The model under review builds one solid part; all positions refer to its coordinate system, in mm. A direction names the side the tool comes from. Coordinates: 2 decimals unless noted, no trailing zeros. Order: outer loops, then holes, each group sorted by start corner. A loop starts at its lowest first (then second) coordinate and runs counter-clockwise, first axis right, second up. Notation, with made-up numbers: M 40.5,12 L 71.5,12 A35 cw 71.5,47 Z; hole C -37,80.25 d7. An arc over 180 degrees is marked long. One line per item, written item: value.
```python
from build123d import *

# Parameters (mm, degrees)
SKETCH_1_W                = 260
SKETCH_1_H                = 220
EXTRUDE_1_DEPTH           = 6
SKETCH_4_W                = 132
SKETCH_4_H                = 134
CUT_EXTRUDE_1_DEPTH       = 171.716138663
HOLE_WIZARD_1_D           = 6.6
HOLE_WIZARD_1_CBORE_D     = 11
HOLE_WIZARD_1_CBORE_DEPTH = 6.8
HOLE_WIZARD_M12_1_D       = 12
CUT_EXTRUDE_2_DEPTH       = 171.716138663
HOLE_WIZARD_M6_1_D        = 5
HOLE_WIZARD_M6_1_DEPTH    = 15
HOLE_WIZARD_M6_1_TIP      = 1.502151548
HOLE_WIZARD_3_D           = 6.6
HOLE_WIZARD_3_CBORE_D     = 11
HOLE_WIZARD_3_CBORE_DEPTH = 87
HOLE_WIZARD_2_D           = 6.6
HOLE_WIZARD_2_CBORE_D     = 11
HOLE_WIZARD_2_CBORE_DEPTH = 48
HOLE_WIZARD_1_2_D         = 4
HOLE_WIZARD_M4_1_D        = 3.3
HOLE_WIZARD_M4_1_DEPTH    = 10.1
HOLE_WIZARD_M4_1_TIP      = 0.991420021
HOLE_WIZARD_M4_2_D        = 3.3
HOLE_WIZARD_M4_2_DEPTH    = 10.1
HOLE_WIZARD_M4_2_TIP      = 0.991420021
CHAMFER_1_SIZE            = 30
FILLET_1_R                = 2


with BuildPart() as part:
    # 草图1 → 凸台-拉伸1 (new, symmetric)
    with BuildSketch(Plane(origin=(0, 0, 0), x_dir=(0, 0, -1), z_dir=(1, 0, 0))):
        Rectangle(SKETCH_1_W, SKETCH_1_H)
    extrude(amount=EXTRUDE_1_DEPTH, both=True)

    # 草图4 → 切除-拉伸1 (cut, through all)
    with BuildSketch(Plane(origin=(6, 0, 0), x_dir=(0, 0, -1), z_dir=(1, 0, 0))):
        with Locations((64, -43)):
            Rectangle(SKETCH_4_W, SKETCH_4_H)
    extrude(amount=-CUT_EXTRUDE_1_DEPTH, mode=Mode.SUBTRACT)

    # Hole Wizard 1 (through all)
    with Locations(Plane(origin=(-6, -19.944864322, 4.622627096), x_dir=(0, 0, -1), z_dir=(-1, 0, 0))):
        with Locations((8.622627096, -106.944864322), (8.622627096, -66.944864322)):
            CounterBoreHole(HOLE_WIZARD_1_D / 2, HOLE_WIZARD_1_CBORE_D / 2, HOLE_WIZARD_1_CBORE_DEPTH)

    # M12 间隙孔1 (through all)
    with Locations(Plane.ZY.offset(6)):
        with Locations((102, 90)):
            Hole(HOLE_WIZARD_M12_1_D / 2)

    # 草图7 → 切除-拉伸2 (cut, through all)
    with BuildSketch(Plane.ZY.offset(6)):
        with BuildLine():
            ThreePointArc((86.666512802, 17.861614446), (96.21364169, 16.477346637), (105.859776773, 16.351071812))
            ThreePointArc((105.859776773, 16.351071812), (112.428311092, 10.436736946), (106.513976226, 3.868202627))
            ThreePointArc((106.513976226, 3.868202627), (95.232902993, 4.015879966), (84.067616667, 5.634769437))
            ThreePointArc((84.067616667, 5.634769437), (79.25364223, 13.047640009), (86.666512802, 17.861614446))
        make_face()
        with BuildLine():
            ThreePointArc((67.434681402, -72.617038622), (88.956175335, -75.737506733), (110.700852725, -76.022160153))
            ThreePointArc((110.700852725, -76.022160153), (116.615187591, -69.453625834), (110.046653272, -63.539290969))
            ThreePointArc((110.046653272, -63.539290969), (89.936914032, -63.276040061), (70.033577537, -60.390193613))
            ThreePointArc((70.033577537, -60.390193613), (62.620706965, -65.20416805), (67.434681402, -72.617038622))
        make_face()
    extrude(amount=-CUT_EXTRUDE_2_DEPTH, mode=Mode.SUBTRACT)

    # M6 螺纹孔1
    with Locations(Plane(origin=(0, 0, -130), x_dir=(-1, 0, 0), z_dir=(0, 0, -1))):
        with Locations((0, 87), (0, 47)):
            Hole(HOLE_WIZARD_M6_1_D / 2, depth=HOLE_WIZARD_M6_1_DEPTH)
            with Locations((0, 0, -(HOLE_WIZARD_M6_1_DEPTH + HOLE_WIZARD_M6_1_TIP / 2))):  # 118° drill point
                Cone(0, HOLE_WIZARD_M6_1_D / 2, HOLE_WIZARD_M6_1_TIP, mode=Mode.SUBTRACT)

    # 打孔尺寸根据内六角圆柱头螺钉的类型3 (through all)
    with Locations(Plane(origin=(4.643601276, 65.309968696, 130), x_dir=(-1, 0, 0), z_dir=(0, 0, 1))):
        with Locations((4.643601276, 75.309968696), (4.643601276, 165.309968696)):
            CounterBoreHole(HOLE_WIZARD_3_D / 2, HOLE_WIZARD_3_CBORE_D / 2, HOLE_WIZARD_3_CBORE_DEPTH)

    # 打孔尺寸根据内六角圆柱头螺钉的类型2 (through all)
    with Locations(Plane(origin=(-2.196087781, 110, 22.857251804), x_dir=(-1, 0, 0), z_dir=(0, 1, 0))):
        with Locations((-2.196087781, -52.857251804), (-2.196087781, -132.857251804)):
            CounterBoreHole(HOLE_WIZARD_2_D / 2, HOLE_WIZARD_2_CBORE_D / 2, HOLE_WIZARD_2_CBORE_DEPTH)

    # Hole Wizard 1 2 (through all)
    with Locations(Plane.ZY.offset(6)):
        with Locations((2, 24)):
            Hole(HOLE_WIZARD_1_2_D / 2)

    # M4 螺纹孔1
    with Locations(Plane.XY.offset(130)):
        with Locations((0, -90), (0, 10)):
            Hole(HOLE_WIZARD_M4_1_D / 2, depth=HOLE_WIZARD_M4_1_DEPTH)
            with Locations((0, 0, -(HOLE_WIZARD_M4_1_DEPTH + HOLE_WIZARD_M4_1_TIP / 2))):  # 118° drill point
                Cone(0, HOLE_WIZARD_M4_1_D / 2, HOLE_WIZARD_M4_1_TIP, mode=Mode.SUBTRACT)

    # M4 螺纹孔2
    with Locations(Plane(origin=(0, 110, 0), x_dir=(1, 0, 0), z_dir=(0, 1, 0))):
        with Locations((0, 80), (0, -80)):
            Hole(HOLE_WIZARD_M4_2_D / 2, depth=HOLE_WIZARD_M4_2_DEPTH)
            with Locations((0, 0, -(HOLE_WIZARD_M4_2_DEPTH + HOLE_WIZARD_M4_2_TIP / 2))):  # 118° drill point
                Cone(0, HOLE_WIZARD_M4_2_D / 2, HOLE_WIZARD_M4_2_TIP, mode=Mode.SUBTRACT)

    # 倒角1
    chamfer_1_edges = [part.edges().sort_by_distance(p)[0] for p in [
        (0, 110, 130),
    ]]
    chamfer(chamfer_1_edges, length=CHAMFER_1_SIZE)

    # 圆角1
    fillet_1_edges = [part.edges().sort_by_distance(p)[0] for p in [
        (0, 80, 130),
        (0, 110, 100),
    ]]
    fillet(fillet_1_edges, radius=FILLET_1_R)


solid = part.part
```
(1) Tool access review of faces 5 (the cylindrical face through (-2.648, 81.547, -3.284)), 6 (the flat face through (0, 62, -114)), 7 (the cylindrical face through (-0.08, -63.3, 90.22)), 8 (the flat face through (0, -96, 43)): name each direction out of +Z, -Z, +X, -X, +Y, -Y from which nothing blocks a thin tool from reaching the whole face with its end or side.
Geometry results:
face 5: -X
face 6: +Y
face 7: +X, -X
face 8: +Z
(2) We need section B-B, the plane z = 40. State the section outline as (x, y) points, plus the area to 3 significant figures.
Geometry results:
outline: M -6,-110 L 6,-110 L 6,110 L -6,110 Z; hole C 0,-100 d6.6; hole C 0,-10 d6.6
area: 2,570 mm2
(3) Mouldability with a two-part tool opening along X and no side actions: class faces 1 (the cylindrical face through (-0.72, -6.78, 22.21)), 2 (the flat face through (0, -45, 2)), 3 (the flat face through (6, 26, 31)), 4 (the flat face through (0.8, 91, -4)) as +X half, -X half, draft (parallel to the pull), parting line (faces both ways), or undercut.
Geometry results:
face 1: undercut
face 2: draft
face 3: +X half
face 4: -X half
(4) For L1, parallel to Y at x = -1.5, z = -4; L2, parallel to Y at x = 0.5, z = 29; L3, parallel to Z at x = 3, y = 96.5, list the stretches that pass through material, from the lowest coordinate up.
Geometry results:
L1: y = 24 to 41.5, 52.5 to 81.5, 92.5 to 110
L2: y = -110 to -103.26, -96.74 to -13.26, -6.74 to 110
L3: z = -130 to -114.61, -105.39 to -34.61, -25.39 to 113.5
(5) We need section D-D, the plane y = -20. State the section outline as (x, z) points, plus the area to 3 significant figures.
Geometry results:
outline: M -6,2 L 6,2 L 6,130 L -6,130 Z
area: 1,540 mm2
(6) We need section C-C, the plane y = 69. State the section outline as (x, z) points, plus the area to 3 significant figures.
Geometry results:
outline: M -6,-130 L 6,-130 L 6,130 L -6,130 Z; hole C 0,-110 d11; hole C 0,-30 d11
area: 2,930 mm2
(7) Insertion check: pin 1 Ø5 at (x, z) = (-4.5, -48) entering from -Y; pin 2 Ø3.5 at (x, z) = (0.5, -111) entering from +Y; pin 3 Ø1.5 at (x, y) = (3.5, 8) entering from -Z; pin 4 Ø3 at (x, y) = (0, 10) entering from +Z. Each pin has a flat end and moves straight along its axis. Give the tip position at first contact, or say it passes through.
Geometry results:
pin 1: stops at y = 24
pin 2: passes through
pin 3: stops at z = 2
pin 4: stops at z = 119.81
(8) We need section A-A, the plane y = -100. State the section outline as (x, z) points.
Geometry results:
outline: M -6,2 L -3.3,2 L -3.3,43 L -5.5,43 L -5.5,130 L -6,130 Z; M 3.3,2 L 6,2 L 6,130 L 5.5,130 L 5.5,43 L 3.3,43 Z
